Autodesk Inventor part; units mm, degrees
ref_plane "YZ Plane" through (0, 0, 0) normal (1, 0, 0) x (0, 1, 0)
ref_plane "XZ Plane" through (0, 0, 0) normal (0, 1, 0) x (-1, 0, 0)
ref_plane "XY Plane" through (0, 0, 0) normal (0, 0, 1) x (1, 0, 0)
sketch "Sketch1" plane through (0, 0, 0) normal (0, 1, 0) x (-1, 0, 0)
  line L0 (-0.4496, -30) -> (-0.4496, 0)
  line L1 (-41.2289, 0) -> (-41.2289, -30)
  circle A0 centre (-20.8393, -15) radius 2.6
  circle A1 centre (-61.4686, -7.475) radius 1.05
  circle A2 centre (-61.4686, -22.525) radius 1.05
  circle A3 centre (-45.8686, -6.93) radius 1.05
  circle A4 centre (-46.3686, -22.525) radius 1.05
  circle A5 centre (4.87, -15) radius 1.05
  circle A6 centre (12.17, -8) radius 1.05
  circle A7 centre (25.39, -7) radius 1.05
  circle A8 centre (12.17, -22) radius 1.05
  circle A9 centre (25.39, -23) radius 1.05
  circle A10 centre (-27.8393, -15) radius 1.05
  circle A11 centre (-20.8393, -8) radius 1.05
  circle A12 centre (-20.8393, -22) radius 1.05
  circle A13 centre (-13.8393, -15) radius 1.05
  arc A14 (-72.2686, -5) -> (-73.2686, -6) centre (-72.2686, -6) ccw
  line L2 (-73.2686, -9.041) -> (-73.2686, -6)
  arc A15 (31.59, -6) -> (30.59, -5) centre (30.59, -6) ccw
  line L3 (31.59, -6) -> (31.59, -9.041)
  arc A16 (30.59, -25) -> (31.59, -24) centre (30.59, -24) ccw
  line L4 (8.19, -25) -> (30.59, -25)
  arc A17 (-73.2686, -24) -> (-72.2686, -25) centre (-72.2686, -24) ccw
  line L5 (-73.2686, -24) -> (-73.2686, -20.959)
  arc A18 (-73.2686, -20.959) -> (-73.2686, -9.041) centre (-73.9686, -15) ccw
  line L6 (-72.2686, -25) -> (-49.8686, -25)
  arc A19 (-49.8686, -25) -> (-44.8686, -30) centre (-44.8686, -25) ccw
  line L7 (3.19, -30) -> (-44.8686, -30)
  arc A20 (3.19, -30) -> (8.19, -25) centre (3.19, -25) ccw
  line L8 (31.59, -20.959) -> (31.59, -24)
  arc A21 (31.59, -9.041) -> (31.59, -20.959) centre (32.29, -15) ccw
  line L9 (30.59, -5) -> (8.19, -5)
  arc A22 (8.19, -5) -> (3.19, 0) centre (3.19, -5) ccw
  line L10 (-44.8686, 0) -> (3.19, 0)
  arc A23 (-44.8686, 0) -> (-49.8686, -5) centre (-44.8686, -5) ccw
  line L11 (-49.8686, -5) -> (-72.2686, -5)
  line L12 (-41.6786, -30) -> (-41.6786, 0)
  line L13 (-40.7793, 0) -> (-40.7793, -30)
  line L14 (-0.8993, -30) -> (-0.8993, 0)
  line L15 (0, 0) -> (0, -30)
extrude "Extrusion1" add sketch "Sketch1" against normal blind 1.5
properties part number "axis_19_top_frame"
Build history of the part. All positions in model axes, mm. Give positions to 0.01 mm unless a question says otherwise; leave off trailing zeros. Loops run counter-clockwise (first coordinate to the right, second up) from the corner with the lowest first, then second, coordinate; pieces in that order, holes last.
1) Two-plate mould, pull along Z, no slides. Class faces 1 (the face through (22, 0, -18)), 2 (the face through (48.37, -0.74, -1.43)), 3 (the face through (21.613, -0.74, -7.29)): released by +Z, released by -Z, zero draft, split by the parting line, or undercut.
Values follow:
face 1: zero draft
face 2: released by +Z
face 3: undercut
2) Band-saw the part on B-B on y = -0.25. State how many separate pieces and enclosed holes the cut face has, then the cut area to 3 significant figures.
Values follow:
separate pieces: 1
enclosed holes: 14
area: 2,490 mm2
3) Drop a flat-ended pin along its axis: P1, Ø0.8, axis at x = 62.5, y = -0.5, coming from the +Z side. Give the stop position or say it passes through.
Values follow:
P1: stops at z = -5
4) Band-saw the part on C-C on z = -10.5. List the corners of the cut face in (x, y), then the cut area to 3 significant figures.
Values follow:
outline: (-28.32, -1.5) - (70, -1.5) - (70, 0) - (-28.32, 0) - close
area: 147 mm2
5) Band-saw the part on A-A on x = -12.17. List the corners of the cut face in (y, z), then the cut area to 3 significant figures.
Values follow:
outline: (-1.5, -25) - (0, -25) - (0, -23.05) - (-1.5, -23.05) - close; (-1.5, -20.95) - (0, -20.95) - (0, -9.05) - (-1.5, -9.05) - close; (-1.5, -6.95) - (0, -6.95) - (0, -5) - (-1.5, -5) - close
area: 23.7 mm2
6) Probe line 1 along Z through (x, y) = (-12.17, -0.9); line 2 along X through (y, z) = (-0.7, -15.5); line 3 along X through (y, z) = (-0.05, -7.75). List the from-to ranges inside material, lowest first.
Values follow:
line 1: z = -25 to -23.05, -20.95 to -9.05, -6.95 to -5
line 2: x = -26.31 to -5.79, -3.95 to 12.92, 14.76 to 18.29, 23.39 to 26.92, 28.76 to 67.99
line 3: x = -31.59 to -26.12, -24.66 to -13.19, -11.15 to 19.82, 21.86 to 45.21, 46.52 to 60.46, 62.48 to 73.27
